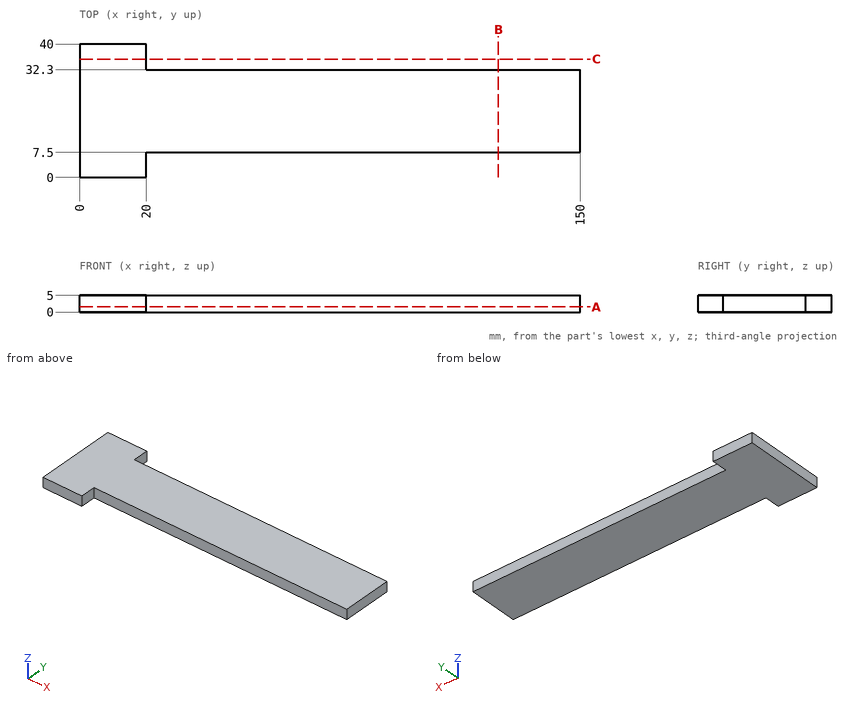
Study the drawing (mm; zero at the part's minimum x, y, z) and answer. Give positions to 0.01 mm unless a question says otherwise; leave off trailing zeros. Order: outer loops, then holes, each group sorted by start corner. A loop starts at its lowest first (then second) coordinate and runs counter-clockwise, first axis right, second up. Notation, with made-up numbers: (20, -8.75) -> (43, -8.75) arc R25 cw to (43, 5.25) -> close; hole circle Ø3 at (2, 1.5). An arc over 180 degrees is marked (long way). Write item = value, one per line.
1. Given pin 1 (2.5 mm diameter, centred on y = 3.5, z = 3, fed in from +X); pin 2 (2.5 mm diameter, centred on x = 110, z = 2.5, fed in from -Y), each flat-ended and moving along its own axis, determine where each tip first touches the part or whether it passes through.
Numbers:
pin_1 = 20
pin_2 = 7.5
2. Straight lines are drawn through the part: line 1 along Y through (x, z) = (62.5, 2.15); line 2 along X through (y, z) = (36, 1.2). For each, find the intervals that lie inside material, in ascending order.
Numbers:
line_1 = 7.5 to 32.3
line_2 = 0 to 20
3. A cutting plane is placed at A-A, the plane z = 1.6. Write down the section's boundary in (x, y).
Numbers:
outline = (0, 0) -> (20, 0) -> (20, 7.5) -> (150, 7.5) -> (150, 32.3) -> (20, 32.3) -> (20, 40) -> (0, 40) -> close
4. A cutting plane is placed at B-B, the plane x = 125.5. Write down the section's boundary in (y, z), and give its area (3 significant figures).
Numbers:
outline = (7.5, 0) -> (32.3, 0) -> (32.3, 5) -> (7.5, 5) -> close
area = 124 mm²
5. A cutting plane is placed at C-C, the plane y = 35.5. Write down the section's boundary in (x, z), and give its area (3 significant figures).
Numbers:
outline = (0, 0) -> (20, 0) -> (20, 5) -> (0, 5) -> close
area = 100 mm²
